from build123d import *

# Parameters (mm, degrees)
BOSS_EXTRUDE1_DEPTH = 5
SKETCH2_R           = 1.95
SKETCH2_W           = 43
SKETCH2_H           = 22
CUT_EXTRUDE1_DEPTH  = 6


with BuildPart() as part:
    # Sketch1 → Boss-Extrude1 (new body)
    with BuildSketch(Plane(origin=(0, 0, 0), x_dir=(1, 0, 0), z_dir=(0, 1, 0))):
        with BuildLine():
            Line((-54, 0), (-2, 0))
            ThreePointArc((-2, 0), (-0.585786438, -0.585786438), (0, -2))
            Line((0, -2), (0, -47.22))
            ThreePointArc((0, -47.22), (-0.585786438, -48.634213562), (-2, -49.22))
            Line((-2, -49.22), (-54, -49.22))
            ThreePointArc((-54, -49.22), (-55.414213562, -48.634213562), (-56, -47.22))
            Line((-56, -47.22), (-56, -2))
            ThreePointArc((-56, -2), (-55.414213562, -0.585786438), (-54, 0))
        make_face()
    extrude(amount=BOSS_EXTRUDE1_DEPTH)

    # Sketch2 → Cut-Extrude1 (cut, through all)
    with BuildSketch(Plane(origin=(0, 5, 0), x_dir=(1, 0, 0), z_dir=(0, 1, 0))):
        with Locations((-4, -4)):
            Circle(SKETCH2_R)
        with Locations((-12, -4)):
            Circle(SKETCH2_R)
        with Locations((18, -4)):
            Circle(SKETCH2_R)
        with Locations((-68, -4)):
            Circle(SKETCH2_R)
        with Locations((-60, -4)):
            Circle(SKETCH2_R)
        with Locations((-52, -4)):
            Circle(SKETCH2_R)
        with Locations((-44, -4)):
            Circle(SKETCH2_R)
        with Locations((-36, -4)):
            Circle(SKETCH2_R)
        with Locations((-28, -4)):
            Circle(SKETCH2_R)
        with Locations((-20, -4)):
            Circle(SKETCH2_R)
        with Locations((-4, -45.22)):
            Circle(SKETCH2_R)
        with Locations((-12, -45.22)):
            Circle(SKETCH2_R)
        with Locations((18, -45.22)):
            Circle(SKETCH2_R)
        with Locations((-68, -45.22)):
            Circle(SKETCH2_R)
        with Locations((-60, -45.22)):
            Circle(SKETCH2_R)
        with Locations((-52, -45.22)):
            Circle(SKETCH2_R)
        with Locations((-44, -45.22)):
            Circle(SKETCH2_R)
        with Locations((-36, -45.22)):
            Circle(SKETCH2_R)
        with Locations((-28, -45.22)):
            Circle(SKETCH2_R)
        with Locations((-20, -45.22)):
            Circle(SKETCH2_R)
        with Locations((-28, -24.61)):
            Rectangle(SKETCH2_W, SKETCH2_H)
    extrude(amount=-CUT_EXTRUDE1_DEPTH, mode=Mode.SUBTRACT)


solid = part.part
Could you check a few things on this model? Use its own coordinates, in mm. A direction names the side the tool comes from. Give positions to 0.01 mm unless a question says otherwise; leave off trailing zeros. Order: outer loops, then holes, each group sorted by start corner. A loop starts at its lowest first (then second) coordinate and runs counter-clockwise, first axis right, second up. Notation, with made-up numbers: (-38, 77.5) -> (-33, 77.5) arc R11 ccw to (-33, 81.5) -> close; hole circle Ø5 at (-36.5, -33.75). An arc over 180 degrees is marked (long way). Answer in a Markdown table with one row per item. Add a question column.
Item 1: Imagine slicing it at C-C (y = 0.8). Count the separate pieces of the cut face and the enclosed holes in it, and give its area (3 significant figures).
Item 2: We'd pull the mould along Z, two halves only. Please class faces 3 (the cylindrical face through (-0.57, 2.46, 48.62)), 4 (the cylindrical face through (-4.423, 2.535, 47.124)), 5 (the flat face through (-28, 5, 13)): pulls with the +Z half, pulls with the -Z half, needs draft (parallel to the pull), parting line crosses it, or undercut.
Item 3: Imagine slicing it at A-A (z = 20). List the corners of the cut face in (x, y) for me.
Item 4: Please list where these lines run through material, in increasing order: probe 1 along Z at (x, y) = (-44, 1.85); probe 2 along Z at (x, y) = (-4, 2.45); probe 3 along X at (y, z) = (4.7, 26).
Item 5: Imagine slicing it at B-B (x = -36). List the corners of the cut face in (y, z) for me, and give its area (3 significant figures).
Item 6: For faces 1 (the cylindrical face through (-0.6, 2.46, 0.57)), 2 (the flat face through (-28, 3, 13.61)), which set-ups out of +Z, -Z, +X, -X, +Y, -Y let a thin tool reach every point of the face, with its end or its side?
Result:
| question | item | result |
|---|---|---|
| 1 | separate pieces | 1 |
| 1 | enclosed holes | 15 |
| 1 | area | 1,640 mm2 |
| 2 | face 3 | pulls with the +Z half |
| 2 | face 4 | undercut |
| 2 | face 5 | needs draft |
| 3 | outline | (-56, 0) -> (-49.5, 0) -> (-49.5, 5) -> (-56, 5) -> close; (-6.5, 0) -> (0, 0) -> (0, 5) -> (-6.5, 5) -> close |
| 4 | probe 1 | 0 to 2.05, 5.95 to 13.61, 35.61 to 43.27, 47.17 to 49.22 |
| 4 | probe 2 | 0 to 2.05, 5.95 to 43.27, 47.17 to 49.22 |
| 4 | probe 3 | -56 to -49.5, -6.5 to 0 |
| 5 | outline | (0, 0) -> (5, 0) -> (5, 2.05) -> (0, 2.05) -> close; (0, 5.95) -> (5, 5.95) -> (5, 13.61) -> (0, 13.61) -> close; (0, 35.61) -> (5, 35.61) -> (5, 43.27) -> (0, 43.27) -> close; (0, 47.17) -> (5, 47.17) -> (5, 49.22) -> (0, 49.22) -> close |
| 5 | area | 97.1 mm2 |
| 6 | face 1 | -Z, +X, +Y, -Y |
| 6 | face 2 | +Y, -Y |
